Verification items for the finished model (mm, model axes). A direction names the side the tool comes from. Coordinates: 2 decimals unless noted, no trailing zeros. Loops run counter-clockwise (first coordinate to the right, second up) from the corner with the lowest first, then second, coordinate; pieces in that order, holes last.
Q1. Sectioned sample at A-A (x = 12.5). Enter the section's corners in (y, z), then the cut area to 3 significant figures.
Q2. Go/stop test with flat-tipped pins: P1, Ø10, axis at y = 7.5, z = 2.5, coming from the -X side; P2, Ø2.5, axis at x = -28.64, y = -2.22, coming from the -Z side; P3, Ø4, axis at x = -32.5, y = 16, coming from the -Z side; P4, Ø3, axis at y = -2.5, z = 13.5, coming from the -X side. Record where each tip stops, or that it passes through.
Q3. Material ranges on probe 1 along Y at (x, z) = (-17, 14); probe 2 along Z at (x, y) = (-30.5, 22.5); probe 3 along Z at (x, y) = (-1, -3), recorded low to high.
Q4. Access from +Z, -Z, +X, -X, +Y, -Y to the whole of each face (thin tool, end or side, straight path). Record for faces 1 (the face through (0, 5.25, 19)), 2 (the face through (3.815, 28.228, 12.799)), 3 (the face through (-3.232, 7.715, 12.099)).
Q5. Mould release check, pull along Y, two halves, no side actions. Record for faces 4 (the face through (0, 17, 16)), 5 (the face through (0, 8, 10.25)), 6 (the face through (-5.37, -7.68, -1.4)): +Y half, -Y half, draft (parallel to the pull), parting line (faces both ways), or undercut.
Q6. Sectioned sample at D-D (y = 3.5). Enter the section's corners in (x, z), then the cut area to 3 significant figures.
Q7. Sectioned sample at C-C (z = 19). Enter the section's corners in (x, y), then the cut area to 3 significant figures.
Q8. Sectioned sample at B-B (x = 0). Enter the section's corners in (y, z).
Autodesk Inventor part; units mm, degrees
ref_plane "YZ Plane" through (0, 0, 0) normal (1, 0, 0) x (0, 1, 0)
ref_plane "XZ Plane" through (0, 0, 0) normal (0, 1, 0) x (-1, 0, 0)
ref_plane "XY Plane" through (0, 0, 0) normal (0, 0, 1) x (1, 0, 0)
sketch "Skizze1" plane through (0, 0, 0) normal (0, 0, 1) x (1, 0, 0)
  line L0 (20.5, -5.25) -> (-20.5, -5.25)
  line L1 (-20.5, -5.25) -> (-20.5, 5.25)
  line L2 (-20.5, 5.25) -> (20.5, 5.25)
  line L3 (20.5, 5.25) -> (20.5, -5.25)
  line L4 (20.5, -5.25) -> (-20.5, 5.25) construction
  line L5 (-20.5, -5.25) -> (20.5, 5.25) construction
  line L6 (-22.5, -8.25) -> (-39.9555, -8.25)
  line L7 (-39.9555, -8.25) -> (-39.9555, 33.1575)
  line L8 (-39.9555, 33.1575) -> (-22.5, 33.1575)
  line L9 (-22.5, 33.1575) -> (-22.5, -8.25)
  line L10 (-22.5, 33.1575) -> (23.5, 33.1575)
  line L11 (23.5, 33.1575) -> (23.5, -8.25)
  line L12 (23.5, -8.25) -> (-22.5, -8.25)
  line L13 (-22.5, -8.25) -> (-22.5, 33.1575)
  line L14 (-22.5, -8.25) -> (-39.9555, -8.25)
  line L15 (-22.5, 30.1575) -> (-39.9555, 30.1575)
  line L16 (-22.5, -8.25) -> (-29.2723, 30.1575)
  line L17 (-32.6543, -8.25) -> (-39.9555, 33.1575)
  line L18 (-36.3049, 12.4538) -> (-25.8861, 10.9538) construction
  line L19 (-34.3494, 30.1575) -> (-27.5771, -8.25) construction
  circle A0 centre (-31.2443, 12.5475) radius 2
  circle A1 centre (-28.6396, -2.2246) radius 2
  line L20 (-29.2723, 30.1575) -> (-39.9555, 28.2738)
  line L21 (-22.5, -8.25) -> (-22.5, -8.25)
  point P0 (0, 0)
  point P1 (-32.6543, -8.25)
  point P2 (-39.4265, 30.1575)
  point P3 (-31.0955, 11.7038)
  point P4 (-39.1204, 28.421)
  point P5 (-32.334, -7.473)
  dimension "d0" = 10.5
  dimension "d1" = 41
  dimension "d2" = 3
  dimension "d3" = 3
  dimension "d4" = 3
  dimension "d6" = 10
  dimension "d7" = 10
  dimension "d16" = 4
  dimension "d18" = 15
  dimension "d21" = 39
  dimension "d23" = 17
  dimension "d24" = 7
  dimension "d29" = 2
extrude "Extrusion1" add sketch "Skizze1" along normal blind 20 contours L16 L15 L9 | L9 L10 L11 L12 | L15 L17 L8 L9 | L20 L17 L15
extrude "Extrusion2" add sketch "Skizze1" against normal blind 2 contours L0 L1 L2 L3 | L16 L15 L9 | L9 L10 L11 L12 | L6 L17 L20 L16 | L15 L17 L8 L9 | L20 L17 L15
sketch "Skizze2" plane through (0, 0, 20) normal (0, 0, 1) x (1, 0, 0)
  line L0 (-39.9555, 33.1575) -> (-39.1204, 28.421)
  line L1 (23.5, -8.25) -> (23.5, 33.1575)
  line L2 (23.5, 33.1575) -> (-39.9555, 33.1575)
  line L3 (20.5, -5.25) -> (-20.5, -5.25)
  line L4 (-20.5, -5.25) -> (-20.5, 5.25)
  line L5 (-20.5, 5.25) -> (20.5, 5.25)
  line L6 (20.5, 5.25) -> (20.5, -5.25)
  line L7 (-39.9555, 33.1575) -> (-32.8306, -7.25)
  line L8 (-39.9555, 33.1575) -> (-32.8306, -7.25)
  circle A0 centre (-28.6396, -2.2246) radius 2
  circle A1 centre (-31.2443, 12.5475) radius 2
  line L9 (-39.1204, 28.421) -> (-29.2723, 30.1575)
  line L10 (-29.2723, 30.1575) -> (-22.5, -8.25)
  line L11 (-22.5, -8.25) -> (23.5, -8.25)
  line L12 (-39.1204, 28.421) -> (-29.2723, 30.1575)
  line L13 (-39.1204, 28.421) -> (-32.6543, -8.25)
  line L14 (-32.6543, -8.25) -> (-22.5, -8.25)
  line L15 (-29.2723, 30.1575) -> (-22.5, -8.25)
  circle A2 centre (-28.6396, -2.2246) radius 2
  circle A3 centre (-31.2443, 12.5475) radius 2
  point P0 (0, 0)
  point P1 (-39.1307, 33.9543)
  point P2 (-39.1307, 33.9543)
  point P3 (-32.6543, -7.25)
  point P4 (-32.8306, -7.25)
extrude "Extrusion3" add sketch "Skizze2" along normal blind 2
fillet "Rundung1" radius 2 9 edges at (-8.2278, 33.1575, 22) (23.5, 12.4538, 22) (23.5, 12.4538, -2) (23.5, 33.1575, 10) (23.5, -8.25, 10) (-4.5771, -8.25, -2) (-8.2278, 33.1575, -2) (-4.5771, -8.25, 22) (-39.9555, 33.1575, 10)
sketch "Skizze3" plane through (-32.6543, -7.5, 20) normal (0, -1, 0) x (1, 0, 0)
  line L0 (53.1543, -20) -> (53.1543, 2)
  line L1 (53.1543, -9) -> (0, -9)
  line L2 (0, -20) -> (0, 0)
  line L3 (53.1543, 2) -> (12.1543, 2)
  line L4 (32.6543, -20) -> (32.6543, 2)
  circle A0 centre (32.6543, -9) radius 2
  dimension "d25" = 4
extrude "Extrusion4" [suppressed]
fillet "Rundung2" [suppressed]
sketch "Skizze5" plane through (-22.5, -8.25, 20) normal (0, -1, 0) x (1, 0, 0)
  line L0 (43, -20) -> (2, -20)
  line L1 (2, -20) -> (2, 2)
  line L2 (43, -20) -> (43, 2)
  line L3 (22.5, -14) -> (22.5, 2) construction
  line L4 (-17.072, 2) -> (44, 2)
  circle A0 centre (22.5, -6) radius 2
  line L5 (43, 2) -> (2, 2)
  line L6 (2, -6) -> (43, -6) construction
  dimension "d34" = 4
  dimension "d45" = 16
extrude "Extrusion6" cut sketch "Skizze5" against normal through all contours A0
fillet "Rundung3" [suppressed]
fillet "Rundung4" radius 3 2 edges at (-33.2443, 12.5475, -2) (-30.6396, -2.2246, -2)
extrude "Extrusion7" add sketch "Skizze5" against normal up to surface (3 mm away) contours A0
sketch "Skizze6" plane through (-37.572, 33.1575, 0) normal (0, 1, 0) x (1, 0, 0)
  circle A0 centre (37.572, -14) radius 2
  circle A1 centre (37.572, -14) radius 2
  circle A2 centre (37.572, -14) radius 4
  point P0 (37.572, 0)
  dimension "d40" = 8
extrude "Extrusion8" cut sketch "Skizze6" against normal blind 10
sketch "Skizze7" plane through (0, 0, 0) normal (0, 0, 1) x (1, 0, 0)
  line L0 (20.5, 5.25) -> (20.5, -5.25)
  line L1 (-20.5, 5.25) -> (20.5, 5.25)
  line L2 (-20.5, -5.25) -> (-20.5, 5.25)
  line L3 (20.5, -5.25) -> (-20.5, -5.25)
  point P0 (0, 0)
extrude "Extrusion9" add sketch "Skizze7" along normal blind 10
sketch "Skizze8" plane through (-20.5, 5.25, 22) normal (0, -1, 0) x (1, 0, 0)
  circle A0 centre (20.5, -8) radius 2
  line L0 (24.8301, -8) -> (22.6651, -11.75)
  line L1 (22.6651, -11.75) -> (18.3349, -11.75)
  line L2 (18.3349, -11.75) -> (16.1699, -8)
  line L3 (16.1699, -8) -> (18.3349, -4.25)
  line L4 (18.3349, -4.25) -> (22.6651, -4.25)
  line L5 (22.6651, -4.25) -> (24.8301, -8)
  line L6 (0, -12) -> (41, -12)
  point P0 (20.5, -22)
  dimension "d46" = 7.5
extrude "Extrusion10" cut sketch "Skizze8" against normal blind 5
equation "\"d3\" = d2"
equation "\"d4\" = d2"
properties part number "_3D-Druck"
Geometry check:
1. outline: (-8.25, 0) arc R2 ccw to (-6.25, -2) - (31.16, -2) arc R2 ccw to (33.16, 0) - (33.16, 20) arc R2 ccw to (31.16, 22) - (5.25, 22) - (5.25, 10) - (-5.25, 10) - (-5.25, 22) - (-6.25, 22) arc R2 ccw to (-8.25, 20) - close
1. area: 864 mm2
2. P1: stops at x = -36.19
2. P2: passes through
2. P3: stops at z = -2
2. P4: stops at x = -23.78
3. probe 1: y = -8.25 to -5.25, 5.25 to 33.16
3. probe 2: z = -2 to 0, 20 to 22
3. probe 3: z = -2 to 10
4. face 1: +Z
4. face 2: +Y
4. face 3: none
5. face 4: draft
5. face 5: undercut
5. face 6: -Y half
6. outline: (-34.73, -2) - (21.5, -2) arc R2 ccw to (23.5, 0) - (23.5, 20) arc R2 ccw to (21.5, 22) - (20.5, 22) - (20.5, 10) - (-20.5, 10) - (-20.5, 22) - (-34.73, 22) - (-34.73, 20) - (-24.57, 20) - (-24.57, 0) - (-34.73, 0) - close
6. area: 701 mm2
7. outline: (-39.54, 30.81) - (-39.12, 28.42) - (-29.27, 30.16) - (-22.5, -8.25) - (21.5, -8.25) arc R2 ccw to (23.5, -6.25) - (23.5, 31.16) arc R2 ccw to (21.5, 33.16) - (-37.57, 33.16) arc R2 ccw to start; hole (-20.5, -5.25) - (20.5, -5.25) - (20.5, 5.25) - (-20.5, 5.25) - close
7. area: 1,660 mm2
8. outline: (-8.25, 0) arc R2 ccw to (-6.25, -2) - (31.16, -2) arc R2 ccw to (33.16, 0) - (33.16, 10) - (23.16, 10) - (23.16, 12) - (10.25, 12) - (10.25, 10.25) - (5.25, 10.25) - (5.25, 10) - (-5.25, 10) - (-5.25, 22) - (-6.25, 22) arc R2 ccw to (-8.25, 20) - close; (5.25, 17.75) - (10.25, 17.75) - (10.25, 16) - (23.16, 16) - (23.16, 18) - (33.16, 18) - (33.16, 20) arc R2 ccw to (31.16, 22) - (5.25, 22) - close
